Part model, mm, in its own coordinate system. Give positions to 0.01 mm unless a question says otherwise; leave off trailing zeros. Order: outer loops, then holes, each group sorted by start corner. A loop starts at its lowest first (then second) coordinate and runs counter-clockwise, first axis right, second up. Notation, with made-up numbers: M 25,56 L 34,56 A34 cw 34,87 Z; hole C 45.5,7 d5. An arc over 180 degrees is marked long. Answer as a JSON object with one key per item and string values.
from build123d import *

# Parameters (mm, degrees)
SKETCH1_R                 = 9.525
BOSS_EXTRUDE1_DEPTH       = 31.75
M6X1_0_TAPPED_HOLE1_D     = 5
M6X1_0_TAPPED_HOLE1_DEPTH = 15.0114
M6X1_0_TAPPED_HOLE1_TIP   = 1.502151548
M6X1_0_TAPPED_HOLE2_D     = 5
M6X1_0_TAPPED_HOLE2_DEPTH = 15.0114
M6X1_0_TAPPED_HOLE2_TIP   = 1.502151548


with BuildPart() as part:
    # Sketch1 → Boss-Extrude1 (new body, symmetric)
    with BuildSketch(Plane.XY):
        Circle(SKETCH1_R)
    extrude(amount=BOSS_EXTRUDE1_DEPTH, both=True)

    # M6x1.0 Tapped Hole1
    with Locations(Plane.XY.offset(31.75)):
        with Locations((0, 0)):
            Hole(M6X1_0_TAPPED_HOLE1_D / 2, depth=M6X1_0_TAPPED_HOLE1_DEPTH)
            with Locations((0, 0, -(M6X1_0_TAPPED_HOLE1_DEPTH + M6X1_0_TAPPED_HOLE1_TIP / 2))):  # 118° drill point
                Cone(0, M6X1_0_TAPPED_HOLE1_D / 2, M6X1_0_TAPPED_HOLE1_TIP, mode=Mode.SUBTRACT)

    # M6x1.0 Tapped Hole2
    with Locations(Plane(origin=(0, 0, -31.75), x_dir=(-1, 0, 0), z_dir=(0, 0, -1))):
        with Locations((0, 0)):
            Hole(M6X1_0_TAPPED_HOLE2_D / 2, depth=M6X1_0_TAPPED_HOLE2_DEPTH)
            with Locations((0, 0, -(M6X1_0_TAPPED_HOLE2_DEPTH + M6X1_0_TAPPED_HOLE2_TIP / 2))):  # 118° drill point
                Cone(0, M6X1_0_TAPPED_HOLE2_D / 2, M6X1_0_TAPPED_HOLE2_TIP, mode=Mode.SUBTRACT)


solid = part.part
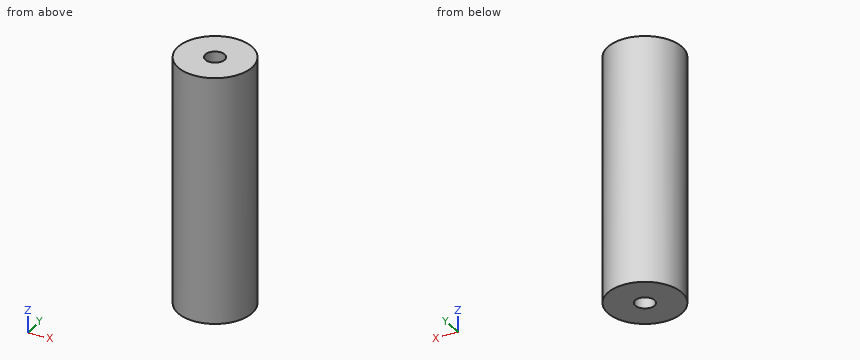
1. Cut at C-C on x = -7.5. Give the cut face in (y, z), plus the area to 3 significant figures.
Worked answers:
{"outline": "M -5.87,-31.75 L 5.87,-31.75 L 5.87,31.75 L -5.87,31.75 Z", "area": "746 mm^2"}
2. Cut at A-A on z = -4. Give the cut face in (x, y) (3 decimals).
Worked answers:
{"outline": "C 0,0 d19.05"}
3. Cut at B-B on y = -6.75. Give the cut face in (x, z), plus the area to 3 significant figures.
Worked answers:
{"outline": "M -6.72,-31.75 L 6.72,-31.75 L 6.72,31.75 L -6.72,31.75 Z", "area": "853 mm^2"}
4. Probe line 1 along Y through (x, z) = (0, -24.5) (3 decimals); line 2 along X through (y, z) = (-0.5, -27); line 3 along X through (y, z) = (-0.5, 7). List the from-to ranges inside material, lowest first.
Worked answers:
{"line 1": "y = -9.525 to -2.5, 2.5 to 9.525", "line 2": "x = -9.51 to -2.45, 2.45 to 9.51", "line 3": "x = -9.51 to 9.51"}
5. Pin check, flat tips, straight feed: P1, Ø4, axis at x = -3, z = -0.5, coming from the -Y side; P2, Ø4, axis at x = 0, y = 0, coming from the +Z side; P3, Ø5, axis at y = 7.5, z = -20, coming from the -X side. Stop position of each tip, or through.
Worked answers:
{"P1": "stops at y = -9.47", "P2": "stops at z = 16.44", "P3": "stops at x = -8.11"}
